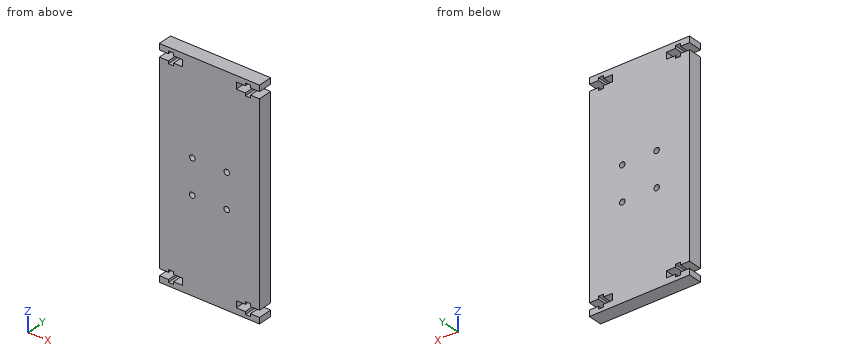
from build123d import *

# Parameters (mm, degrees)
F0_R     = 1.25
F1_DEPTH = 6.35


with BuildPart() as f1:
    # F0 (on Front) → F1 (new body)
    with BuildSketch(Plane.XZ):
        Polygon((22.625, 47.26), (22.625, 50), (-22.625, 50), (-22.625, 47.26), (-18.545, 47.26), (-18.545, 48.465), (-16.205, 48.465), (-16.205, 47.26), (-12.125, 47.26), (-12.125, 44.26), (-16.205, 44.26), (-16.205, 43.055), (-18.545, 43.055), (-18.545, 44.26), (-22.625, 44.26), (-22.625, -44.26), (-18.545, -44.26), (-18.545, -43.055), (-16.205, -43.055), (-16.205, -44.26), (-12.125, -44.26), (-12.125, -47.26), (-16.205, -47.26), (-16.205, -48.465), (-18.545, -48.465), (-18.545, -47.26), (-22.625, -47.26), (-22.625, -50), (22.625, -50), (22.625, -47.26), (18.545, -47.26), (18.545, -48.465), (16.205, -48.465), (16.205, -47.26), (12.125, -47.26), (12.125, -44.26), (16.205, -44.26), (16.205, -43.055), (18.545, -43.055), (18.545, -44.26), (22.625, -44.26), (22.625, 44.26), (18.545, 44.26), (18.545, 43.055), (16.205, 43.055), (16.205, 44.26), (12.125, 44.26), (12.125, 47.26), (16.205, 47.26), (16.205, 48.465), (18.545, 48.465), (18.545, 47.26), align=None)
        with Locations((-7.778175, -7.778175)):
            Circle(F0_R, mode=Mode.SUBTRACT)
        with Locations((7.778175, -7.778175)):
            Circle(F0_R, mode=Mode.SUBTRACT)
        with Locations((-7.778175, 7.778175)):
            Circle(F0_R, mode=Mode.SUBTRACT)
        with Locations((7.778175, 7.778175)):
            Circle(F0_R, mode=Mode.SUBTRACT)
    extrude(amount=F1_DEPTH)


solid = f1.part
Read the model definition and answer for the solid it produces. Units are mm, in the model's axes. Round coordinates to 2 decimals unless told otherwise and drop trailing zeros. Order: outer loops, then holes, each group sorted by start corner. A loop starts at its lowest first (then second) coordinate and runs counter-clockwise, first axis right, second up. Notation, with made-up numbers: (10.5, 27.5) - (36.5, 27.5) arc R26 cw to (36.5, 43.5) - close; hole circle Ø11 at (47.5, 82.5). An arc over 180 degrees is marked (long way). Use one line per item in the form item = value. Start each with the question number.
(1) The part is cut by section A-A (x = 19.5). Give the vertices of the cut face in (y, z).
(2) A flat-ended cylindrical pin translates along its axis: pin 1 Ø3.5 at (y, z) = (-2, 45) entering from +X (3 decimals). Find the tip coordinate at first contact, or state that the pin passes through.
(3) Find the intervals of material crossed by line 1 along Z through (x, y) = (17, -5.5) (3 decimals); line 2 along Z through (x, y) = (15, -5); line 3 along X through (y, z) = (-4, -8) (3 decimals), in increasing order. Write a range as from..to.
(4) The part is cut by section B-B (y = -1.25). Count the separate pieces of the cut face and the enclosed holes in it, then the cut area to 3 significant figures.
Checked values:
q1.outline = (-6.35, -50) - (0, -50) - (0, -47.26) - (-6.35, -47.26) - close; (-6.35, -44.26) - (0, -44.26) - (0, 44.26) - (-6.35, 44.26) - close; (-6.35, 47.26) - (0, 47.26) - (0, 50) - (-6.35, 50) - close
q2.pin_1 = 22.625
q3.line_1 = -50..-48.465, -43.055..43.055, 48.465..50
q3.line_2 = -50..-47.26, -44.26..44.26, 47.26..50
q3.line_3 = -22.625..-9.008, -6.548..6.548, 9.008..22.625
q4.separate_pieces = 1
q4.enclosed_holes = 4
q4.area = 4,360 mm^2
